Could you check a few things on this model? Use its own coordinates, in mm. A direction names the side the tool comes from. Give positions to 0.01 mm unless a question says otherwise; leave off trailing zeros. Write each loop counter-clockwise with the first axis right and the second up, starting at its lowest first coordinate (ties: lowest second). Pieces come first, ordered by that corner, then holes. Notation, with made-up numbers: M -37.75,22 L -26.75,22 A9 cw -26.75,33 Z; hole C 65.25,8 d11. An arc over 180 degrees is marked long. Use one line per item in the form item = value.
from build123d import *

# Parameters (mm, degrees)
MOTOR_SHELL_DEPTH                   = 33.6
MOTOR_MOUNT_DEPTH                   = 4
MOUNTING_HOLE_D                     = 3.6
MOUNTING_HOLE_CSINK_D               = 7.72
MOUNTING_HOLE_CSINK_ANGLE           = 90
HOLE_DUPLICATION_COUNT              = 3
SKETCH11_R                          = 6.5
SHAFT_BASE_CUTOUT_DEPTH             = 34.6
CSK_FOR_M3_INSERT_SFHCS1_AT_2_COUNT = 2
CSK_FOR_M3_INSERT_SFHCS1_AT_2_PITCH = 20
CSK_FOR_M3_INSERT_SFHCS1_AT_3_COUNT = 2
CSK_FOR_M3_INSERT_SFHCS1_AT_3_PITCH = 43.289721644
CSK_FOR_M3_INSERT_SFHCS1_AT_4_COUNT = 2
CSK_FOR_M3_INSERT_SFHCS1_AT_4_PITCH = 48.301138703
CSK_FOR_M3_INSERT_SFHCS2_AT_2_COUNT = 2
CSK_FOR_M3_INSERT_SFHCS2_AT_2_PITCH = 14
CSK_FOR_M3_INSERT_SFHCS2_AT_3_COUNT = 2
CSK_FOR_M3_INSERT_SFHCS2_AT_3_PITCH = 26.925824036
CSK_FOR_M3_INSERT_SFHCS2_AT_4_COUNT = 2
CSK_FOR_M3_INSERT_SFHCS2_AT_4_PITCH = 23
CUT_EXTRUDE1_DEPTH                  = 29.6
CSK_FOR_M3_INSERT_SFHCS3_AT_2_COUNT = 2
CSK_FOR_M3_INSERT_SFHCS3_AT_2_PITCH = 14
CSK_FOR_M3_INSERT_SFHCS3_AT_3_COUNT = 2
CSK_FOR_M3_INSERT_SFHCS3_AT_3_PITCH = 26.925824036
CSK_FOR_M3_INSERT_SFHCS3_AT_4_COUNT = 2
CSK_FOR_M3_INSERT_SFHCS3_AT_4_PITCH = 23
ADDITIONAL_STRUCTURE_DEPTH          = 2


with BuildPart() as part:
    # Motor Shell Profile → Motor Shell (new body)
    with BuildSketch(Plane(origin=(0, 0, 0), x_dir=(0, 0, -1), z_dir=(1, 0, 0))):
        with BuildLine():
            Line((0, 22), (-16, 22))
            Line((-16, 22), (-16, 27.5))
            Line((-16, 27.5), (18, 27.5))
            Line((18, 27.5), (24.57187505, 8.498409058))
            ThreePointArc((24.57187505, 8.498409058), (25.476909304, -5.189132134), (19.290322581, -17.432253289))
            ThreePointArc((19.290322581, -17.432253289), (18.333717374, -18.988556671), (18, -20.784609691))
            Line((18, -20.784609691), (18, -29))
            Line((18, -29), (-16, -29))
            Line((-16, -29), (-16, -22))
            Line((-16, -22), (0, -22))
            ThreePointArc((0, -22), (22, 0), (0, 22))
        make_face()
    extrude(amount=MOTOR_SHELL_DEPTH)

    # Sketch3 → Motor Mount (add)
    with BuildSketch(Plane(origin=(29.6, 0, 0), x_dir=(0, 0, -1), z_dir=(1, 0, 0))):
        with BuildLine():
            Line((0, 22), (-16, 22))
            Line((-16, 22), (-16, -22))
            Line((-16, -22), (0, -22))
            ThreePointArc((0, -22), (22, 0), (0, 22))
        make_face()
    extrude(amount=MOTOR_MOUNT_DEPTH)

    # Mounting Hole (through all)
    with Locations(Plane(origin=(33.6, 0, 0), x_dir=(0, 0, -1), z_dir=(1, 0, 0))):
        with Locations((10.573878655, -3.032010914)):
            mounting_hole = CounterSinkHole(MOUNTING_HOLE_D / 2, MOUNTING_HOLE_CSINK_D / 2, counter_sink_angle=MOUNTING_HOLE_CSINK_ANGLE)

    # Hole Duplication: Mounting Hole ×3 about axis
    hole_duplication_axis = Axis((0, 0, 0), (1, 0, 0))
    for i in range(1, HOLE_DUPLICATION_COUNT):
        add(mounting_hole.rotate(hole_duplication_axis, i * 360 / HOLE_DUPLICATION_COUNT), mode=Mode.SUBTRACT)

    # Sketch11 → Shaft Base Cutout (cut, through all)
    with BuildSketch(Plane(origin=(33.6, 0, 0), x_dir=(0, 0, -1), z_dir=(1, 0, 0))):
        Circle(SKETCH11_R)
    extrude(amount=-SHAFT_BASE_CUTOUT_DEPTH, mode=Mode.SUBTRACT)

    # Sketch15 → CSK for M3 Insert SFHCS1 (revolve, cut)
    with BuildSketch(Plane(origin=(33.6, -25, 7), x_dir=(0, 0, -1), z_dir=(0, 1, 0))):
        Polygon((0, 0), (0, 3.8), (2.55, 3.8), (2.55, 1.501569957), (2.655, 0), align=None)
    csk_for_m3_insert_sfhcs1 = revolve(axis=Axis((39.95, -25, 7), (-1, 0, 0)), mode=Mode.SUBTRACT)

    # CSK for M3 Insert SFHCS1 at 2: CSK for M3 Insert SFHCS1 ×2
    with Locations(*[(0, 0, -i * CSK_FOR_M3_INSERT_SFHCS1_AT_2_PITCH) for i in range(1, CSK_FOR_M3_INSERT_SFHCS1_AT_2_COUNT)]):
        add(csk_for_m3_insert_sfhcs1, mode=Mode.SUBTRACT)

    # CSK for M3 Insert SFHCS1 at 3: CSK for M3 Insert SFHCS1 ×2
    with Locations(*[Vector(0, 0.99330738, 0.115500858) * (i * CSK_FOR_M3_INSERT_SFHCS1_AT_3_PITCH) for i in range(1, CSK_FOR_M3_INSERT_SFHCS1_AT_3_COUNT)]):
        add(csk_for_m3_insert_sfhcs1, mode=Mode.SUBTRACT)

    # CSK for M3 Insert SFHCS1 at 4: CSK for M3 Insert SFHCS1 ×2
    with Locations(*[Vector(0, 0.890248163, -0.455475804) * (i * CSK_FOR_M3_INSERT_SFHCS1_AT_4_PITCH) for i in range(1, CSK_FOR_M3_INSERT_SFHCS1_AT_4_COUNT)]):
        add(csk_for_m3_insert_sfhcs1, mode=Mode.SUBTRACT)

    # Sketch18 → CSK for M3 Insert SFHCS2 (revolve, cut)
    with BuildSketch(Plane(origin=(22, 27.5, 12), x_dir=(0, 0, 1), z_dir=(1, 0, 0))):
        Polygon((0, 0), (0, 3.8), (2.55, 3.8), (2.55, 1.501569957), (2.655, 0), align=None)
    csk_for_m3_insert_sfhcs2 = revolve(axis=Axis((22, 33.85, 12), (0, -1, 0)), mode=Mode.SUBTRACT)

    # CSK for M3 Insert SFHCS2 at 2: CSK for M3 Insert SFHCS2 ×2
    with Locations(*[(-i * CSK_FOR_M3_INSERT_SFHCS2_AT_2_PITCH, 0, 0) for i in range(1, CSK_FOR_M3_INSERT_SFHCS2_AT_2_COUNT)]):
        add(csk_for_m3_insert_sfhcs2, mode=Mode.SUBTRACT)

    # CSK for M3 Insert SFHCS2 at 3: CSK for M3 Insert SFHCS2 ×2
    with Locations(*[Vector(-0.519946947, 0, -0.854198556) * (i * CSK_FOR_M3_INSERT_SFHCS2_AT_3_PITCH) for i in range(1, CSK_FOR_M3_INSERT_SFHCS2_AT_3_COUNT)]):
        add(csk_for_m3_insert_sfhcs2, mode=Mode.SUBTRACT)

    # CSK for M3 Insert SFHCS2 at 4: CSK for M3 Insert SFHCS2 ×2
    with Locations(*[(0, 0, -i * CSK_FOR_M3_INSERT_SFHCS2_AT_4_PITCH) for i in range(1, CSK_FOR_M3_INSERT_SFHCS2_AT_4_COUNT)]):
        add(csk_for_m3_insert_sfhcs2, mode=Mode.SUBTRACT)

    # Sketch25 → Cut-Extrude1 (cut)
    with BuildSketch(Plane.ZY):
        with BuildLine():
            Line((0, 23), (16, 23))
            Line((16, 23), (16, -23))
            Line((16, -23), (0, -23))
            ThreePointArc((0, -23), (-23, 0), (0, 23))
        make_face()
    extrude(amount=-CUT_EXTRUDE1_DEPTH, mode=Mode.SUBTRACT)

    # Sketch27 → CSK for M3 Insert SFHCS3 (revolve, cut)
    with BuildSketch(Plane(origin=(8, -29, 12), x_dir=(0, 0, -1), z_dir=(1, 0, 0))):
        Polygon((0, 0), (0, 3.8), (2.55, 3.8), (2.55, 1.501569957), (2.655, 0), align=None)
    csk_for_m3_insert_sfhcs3 = revolve(axis=Axis((8, -35.35, 12), (0, 1, 0)), mode=Mode.SUBTRACT)

    # CSK for M3 Insert SFHCS3 at 2: CSK for M3 Insert SFHCS3 ×2
    with Locations(*[(i * CSK_FOR_M3_INSERT_SFHCS3_AT_2_PITCH, 0, 0) for i in range(1, CSK_FOR_M3_INSERT_SFHCS3_AT_2_COUNT)]):
        add(csk_for_m3_insert_sfhcs3, mode=Mode.SUBTRACT)

    # CSK for M3 Insert SFHCS3 at 3: CSK for M3 Insert SFHCS3 ×2
    with Locations(*[Vector(0.519946947, 0, -0.854198556) * (i * CSK_FOR_M3_INSERT_SFHCS3_AT_3_PITCH) for i in range(1, CSK_FOR_M3_INSERT_SFHCS3_AT_3_COUNT)]):
        add(csk_for_m3_insert_sfhcs3, mode=Mode.SUBTRACT)

    # CSK for M3 Insert SFHCS3 at 4: CSK for M3 Insert SFHCS3 ×2
    with Locations(*[(0, 0, -i * CSK_FOR_M3_INSERT_SFHCS3_AT_4_PITCH) for i in range(1, CSK_FOR_M3_INSERT_SFHCS3_AT_4_COUNT)]):
        add(csk_for_m3_insert_sfhcs3, mode=Mode.SUBTRACT)

    # Sketch30 → Additional structure (add)
    with BuildSketch(Plane.XY.offset(16)):
        Polygon((0, 23), (29.6, 23), (29.6, -23), (0, -23), (0, -29), (33.6, -29), (33.6, 27.5), (0, 27.5), align=None)
    extrude(amount=ADDITIONAL_STRUCTURE_DEPTH)


solid = part.part
1) For faces 1 (the cylindrical face through (30.56, -6.42, 6.59)), 2 (the cylindrical face through (23.552, 24.865, 9.976)), 3 (the cylindrical face through (9.552, -26.365, 14.024)), 4 (the flat face through (15, -23, 9)), 5 (the conical face through (32.69, 20.53, -14.44)), which set-ups out of +Z, -Z, +X, -X, +Y, -Y let a thin tool reach every point of the face, with its end or its side?
Checked values:
face_1 = +X, -X
face_2 = +Y
face_3 = -Y
face_4 = +Z, -X
face_5 = +X
2) For pin 1 Ø3 at (x, z) = (8, 12) entering from +Y; pin 2 Ø4 at (y, z) = (18, 12) entering from +X; pin 3 Ø3 at (y, z) = (-3.03, -10.57) entering from -X; pin 4 Ø1.5 at (x, y) = (6, 3) entering from -Z, each with a flat end and sliding along its axis, tell me the tip position at first contact or that it passes through.
Checked values:
pin_1 = 23.7
pin_2 = 29.8
pin_3 = through
pin_4 = -25.9
3) I want a section at D-D, the plane y = 18. Please give me the cut outline in (x, z) (3 decimals), plus the area to 3 significant figures.
Checked values:
outline = M 0,-21.286 L 33.6,-21.286 L 33.6,-17.655 L 32.098,-17.55 L 29.8,-17.55 L 29.8,-12.45 L 32.098,-12.45 L 33.6,-12.345 L 33.6,9.345 L 32.098,9.45 L 29.8,9.45 L 29.8,14.55 L 32.098,14.55 L 33.6,14.655 L 33.6,18 L 29.6,18 L 29.6,-14.318 L 0,-14.318 Z
area = 324 mm2
4) I want a section at B-B, the plane x = 16. Please give me the cut outline in (y, z).
Checked values:
outline = M -29,-18 L -20.78,-18 A5 cw -17.43,-19.29 A26 ccw 8.5,-24.57 L 27.5,-18 L 27.5,18 L 23,18 L 23,0 A23 cw -23,0 L -23,18 L -29,18 Z
5) I want a section at A-A, the plane y = 1.5. Please give me the cut outline in (x, z).
Checked values:
outline = M 0,-25.96 L 33.6,-25.96 L 33.6,-6.32 L 29.6,-6.32 L 29.6,-22.95 L 0,-22.95 Z; M 29.6,6.32 L 33.6,6.32 L 33.6,18 L 29.6,18 Z
6) I want a section at C-C, the plane x = 30.5. Count the separate pieces of the cut face and the enclosed holes in it, plus the area to 3 significant figures.
Checked values:
separate_pieces = 1
enclosed_holes = 8
area = 2,020 mm2
7) Thinking about a two-plate mould opening in Y: for faces 6 (the flat face through (8, 23.7, 12)), 7 (the flat face through (29.8, -25, 7)), 8 (the cylindrical face through (16.565, -4.999, -25.515)), which applies, released by +Y, released by -Y, zero draft, split by the parting line, or undercut?
Checked values:
face_6 = released by +Y
face_7 = undercut
face_8 = split by the parting line
8) If I drill on L1, parallel to X at y = -26, z = 12; L2, parallel to Z at x = 30.5, y = -25; L3, parallel to Y at x = 4, z = 5, over which ranges is the centre line in solid material (lowest first)?
Checked values:
L1 = 0 to 5.45, 10.55 to 19.45, 24.55 to 33.6
L2 = -18 to -15.55, -10.45 to 4.45, 9.55 to 18
L3 = -29 to -23, 23 to 27.5
